Here's how the part is built. I have some questions about the finished solid (model axes, mm). A direction names the side the tool comes from. Give positions to 0.01 mm unless a question says otherwise; leave off trailing zeros. Loops run counter-clockwise (first coordinate to the right, second up) from the corner with the lowest first, then second, coordinate; pieces in that order, holes last. Notation, with made-up numbers: (-38.75, -31) - (-9.75, -31) arc R14 ccw to (-9.75, -12) - close; hole circle Ø5 at (-38, -18). An arc over 180 degrees is marked (long way). Use one line per item in the form item = value.
from build123d import *

# Parameters (mm, degrees)
SKETCH1_W           = 85
SKETCH1_H           = 10
SKETCH1_R           = 2
BOSS_EXTRUDE1_DEPTH = 2
CUT_EXTRUDE1_DEPTH  = 10
SKETCH3_W           = 15
SKETCH3_H           = 10
BOSS_EXTRUDE2_DEPTH = 13
BOSS_EXTRUDE3_DEPTH = 10


with BuildPart() as part:
    # Sketch1 → Boss-Extrude1 (new body)
    with BuildSketch(Plane(origin=(0, 0, 0), x_dir=(1, 0, 0), z_dir=(0, 1, 0))):
        with Locations((18.270818553, 2.053936679)):
            Rectangle(SKETCH1_W, SKETCH1_H)
        with Locations(Location((-19.229181447, 2.053936679, 0), (0, 0, 270))):
            Circle(SKETCH1_R, mode=Mode.SUBTRACT)
        with Locations(Location((5.770818553, 2.053936679, 0), (0, 0, 270))):
            Circle(SKETCH1_R, mode=Mode.SUBTRACT)
    extrude(amount=BOSS_EXTRUDE1_DEPTH)

    # Sketch2 → Cut-Extrude1 (cut)
    with BuildSketch(Plane(origin=(0, 2, 0), x_dir=(1, 0, 0), z_dir=(0, 1, 0))):
        Polygon((60.770818553, 2.053936679), (55.770818553, -2.946063321), (60.770818553, -2.946063321), align=None)
    extrude(amount=-CUT_EXTRUDE1_DEPTH, mode=Mode.SUBTRACT)

    # Sketch3 → Boss-Extrude2 (add)
    with BuildSketch(Plane(origin=(29.358440937, 0, 29.358440937), x_dir=(0.7071067811865439, 0, -0.7071067811865511), z_dir=(0.7071067811865511, 0, 0.7071067811865439))):
        with Locations((38.590339713, 0.888307249)):
            Rectangle(SKETCH3_W, SKETCH3_H)
    extrude(amount=BOSS_EXTRUDE2_DEPTH)

    # Sketch4 → Boss-Extrude3 (add)
    with BuildSketch(Plane(origin=(0, 5.888307249, 0), x_dir=(1, 0, 0), z_dir=(0, 1, 0))):
        Polygon((51.342630977, -7.374250897), (49.762527896, -2.752596668), (55.964285206, -2.752596668), align=None)
    extrude(amount=-BOSS_EXTRUDE3_DEPTH)


solid = part.part
(1) For faces 4 (the flat face through (12, 1, 2.946)), 5 (the flat face through (61, -4.112, 7)), 6 (the flat face through (53, -2, 2.753)), which set-ups out of +Z, -Z, +X, -X, +Y, -Y let a thin tool reach every point of the face, with its end or its side?
Geometry says:
face_4 = +Z, -X, +Y, -Y
face_5 = +Z, -Z, +X, -X, -Y
face_6 = -Z, -X, -Y
(2) If I drill on probe 1 along Y at (x, z) = (24.5, -1); probe 2 along Z at (x, y) = (14, 0.5); probe 3 along X at (y, z) = (1.75, -6), over which ranges is the centre line in solid material (lowest first)?
Geometry says:
probe_1 = 0 to 2
probe_2 = -7.05 to 2.95
probe_3 = -24.23 to 60.77
(3) If we section it at B-B (y = -1.75): List the corners of the cut face in (x, z) for me.
Geometry says:
outline = (49.76, 2.75) - (55.96, 2.75) - (61.95, -3.23) - (71.14, 5.96) - (60.54, 16.57) - (51.34, 7.37) - close
(4) Thinking about a two-plate mould opening in Z: for faces 1 (the flat face through (-24.229, 1, -2)), 2 (the cylindrical face through (4.55, 0.99, -3.64)), 3 (the flat face through (53, 4, 2.753)), which applies, pulls with the +Z half, pulls with the -Z half, needs draft (parallel to the pull), parting line crosses it, or undercut?
Geometry says:
face_1 = needs draft
face_2 = undercut
face_3 = pulls with the -Z half
(5) If we section it at D-D (x = 34.5): List the corners of the cut face in (y, z) for me.
Geometry says:
outline = (0, -7.05) - (2, -7.05) - (2, 2.95) - (0, 2.95) - close
(6) If we section it at A-A (x = 52.5): List the corners of the cut face in (y, z) for me, plus the area to 3 significant figures.
Geometry says:
outline = (-4.11, 2.75) - (0, 2.75) - (0, -7.05) - (2, -7.05) - (2, 2.75) - (5.89, 2.75) - (5.89, 8.53) - (-4.11, 8.53) - close
area = 77.4 mm²
(7) If we section it at C-C (z = 11.5): List the corners of the cut face in (x, y) for me, plus the area to 3 significant figures.
Geometry says:
outline = (55.47, -4.11) - (65.6, -4.11) - (65.6, 5.89) - (55.47, 5.89) - close
area = 101 mm²
(8) For P1, Ø2, axis at x = 51.5, y = -3, coming from the -Z side; P2, Ø3, axis at x = 40, z = 1, coming from the +Y side; P3, Ø11, axis at x = 24, z = -2.5, coming from the -Y side; P4, Ø3.5, axis at x = 5.77, z = -2.05, coming from the -Y side, each with a flat end and sliding along its axis, tell me the tip position at first contact or that it passes through.
Geometry says:
P1 = 2.75
P2 = 2
P3 = 0
P4 = through
